Input: part model. Units: mm. Frame: model coordinates. Face numbers are marked on the shaded views. Give positions to 0.01 mm unless a question says otherwise; leave off trailing zeros. Loops run counter-clockwise (first coordinate to the right, second up) from the corner with the lowest first, then second, coordinate; pieces in that order, holes last. Notation, with made-up numbers: (-16, 13.5) -> (-10, 13.5) arc R17 ccw to (-10, 31.5) -> close; hole circle Ø5 at (19, 55.5). An arc over 180 degrees is marked (long way). Use CSV: the item, a comma, the result in double quotes.
```python
from build123d import *

# Parameters (mm, degrees)
SKETCH_1_R               = 350
EXTRUDE_1_DEPTH          = 200
SKETCH_2_R               = 210
EXTRUDE_2_DEPTH          = 300
SKETCH_3_R               = 340
SKETCH_3_R_2             = 244
CUT_EXTRUDE_1_DEPTH      = 2
SKETCH_4_R               = 25
CUT_EXTRUDE_2_DEPTH      = 704.562363974
PATTERN_CIRCULAR_1_COUNT = 8


with BuildPart() as part:
    # 草图1 → 凸台-拉伸1 (new body)
    with BuildSketch(Plane.XY):
        Circle(SKETCH_1_R)
    extrude(amount=EXTRUDE_1_DEPTH)

    # 草图2 → 凸台-拉伸2 (add)
    with BuildSketch(Plane.XY.offset(200)):
        Circle(SKETCH_2_R)
    extrude(amount=EXTRUDE_2_DEPTH)

    # 草图3 → 切除-拉伸1 (cut)
    with BuildSketch(Plane.XY.offset(200)):
        Circle(SKETCH_3_R)
        Circle(SKETCH_3_R_2, mode=Mode.SUBTRACT)
    extrude(amount=-CUT_EXTRUDE_1_DEPTH, mode=Mode.SUBTRACT)

    # 草图4 → 切除-拉伸2 (cut, through all)
    with BuildSketch(Plane(origin=(0, 0, 0), x_dir=(-1, 0, 0), z_dir=(0, 0, -1))):
        with Locations((0, 290)):
            Circle(SKETCH_4_R)
    cut_extrude_2 = extrude(amount=-CUT_EXTRUDE_2_DEPTH, mode=Mode.SUBTRACT)

    # 阵列(圆周)1: 切除-拉伸2 ×8 about axis
    pattern_circular_1_axis = Axis((0, 0, 0), (0, 0, 1))
    for i in range(1, PATTERN_CIRCULAR_1_COUNT):
        add(cut_extrude_2.rotate(pattern_circular_1_axis, i * 360 / PATTERN_CIRCULAR_1_COUNT), mode=Mode.SUBTRACT)


solid = part.part
```
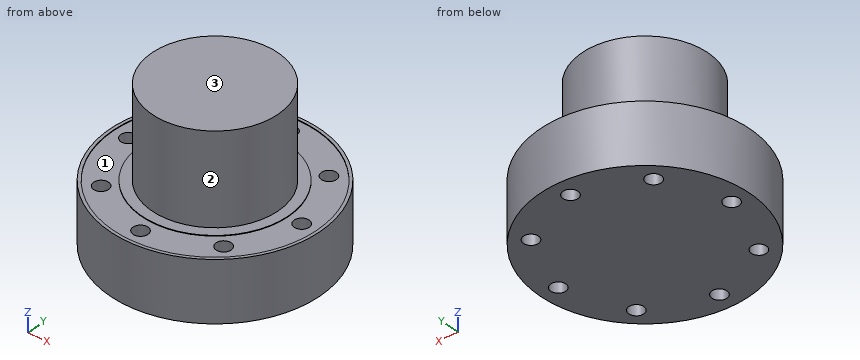
1) Mould query, pull axis Y, two halves, no side actions, for the marked faces 1, 2 and 3. Classes: pulls with the +Y half, pulls with the -Y half, needs draft (parallel to the pull), parting line crosses it, or undercut.
From the geometry:
face 1,"undercut"
face 2,"parting line crosses it"
face 3,"needs draft"
2) Ray query, line 1 (Y direction, x = -183, z = 63); line 2 (Z direction, x = 228, y = 133); line 3 (Z direction, x = 68, y = -221). Return the intervals inside material, ascending.
From the geometry:
line 1,"y = -298.35 to -216.82, -193.3 to 193.3, 216.82 to 298.35"
line 2,"z = 0 to 198"
line 3,"z = 0 to 200"
3) Section query C-C (y = 76.5). Return loops of the section in (x, z).
From the geometry:
outline,"(-341.54, 0) -> (341.54, 0) -> (341.54, 200) -> (331.28, 200) -> (331.28, 198) -> (231.7, 198) -> (231.7, 200) -> (195.57, 200) -> (195.57, 500) -> (-195.57, 500) -> (-195.57, 200) -> (-231.7, 200) -> (-231.7, 198) -> (-331.28, 198) -> (-331.28, 200) -> (-341.54, 200) -> close"
4) Section query A-A (y = 0). Return loops of the section in (x, z).
From the geometry:
outline,"(-350, 0) -> (-315, 0) -> (-315, 198) -> (-340, 198) -> (-340, 200) -> (-350, 200) -> close; (-265, 0) -> (265, 0) -> (265, 198) -> (244, 198) -> (244, 200) -> (210, 200) -> (210, 500) -> (-210, 500) -> (-210, 200) -> (-244, 200) -> (-244, 198) -> (-265, 198) -> close; (315, 0) -> (350, 0) -> (350, 200) -> (340, 200) -> (340, 198) -> (315, 198) -> close"
5) Contact query for flat-ended pins moving along their axis: pin 1 (10 mm diameter, centred on x = 225, y = 4.5, fed in from -Z); pin 2 (3 mm diameter, centred on y = -238.5, z = 174.5, fed in from +X); pin 3 (1 mm diameter, centred on y = -129, z = 334.5, fed in from -X); pin 4 (6 mm diameter, centred on y = 96, z = 148.5, fed in from -X). Output: stop coordinate, or through.
From the geometry:
pin 1,"stops at z = 0"
pin 2,"stops at x = 257.55"
pin 3,"stops at x = -166.1"
pin 4,"stops at x = -337.42"
6) Section query D-D (x = 290). Return loops of the section in (y, z), then the cut area to 3 significant figures.
From the geometry:
outline,"(-195.96, 0) -> (-25, 0) -> (-25, 198) -> (-177.48, 198) -> (-177.48, 200) -> (-195.96, 200) -> close; (25, 0) -> (195.96, 0) -> (195.96, 200) -> (177.48, 200) -> (177.48, 198) -> (25, 198) -> close"
area,"67,800 mm^2"
